Drawing for the job (mm, zero at the part's lowest x, y, z). A direction names the side the tool comes from. Round coordinates to 2 decimals unless told otherwise and drop trailing zeros. Write each loop counter-clockwise with the first axis right and the second up, starting at its lowest first coordinate (ties: lowest second). Pieces come first, ordered by that corner, then holes. Notation, with made-up numbers: (16.5, 46) -> (24.5, 46) arc R15 ccw to (24.5, 75) -> close; hole circle Ø5 at (63.25, 53.25). An arc over 180 degrees is marked (long way). One line per question, with ' | ' between items.
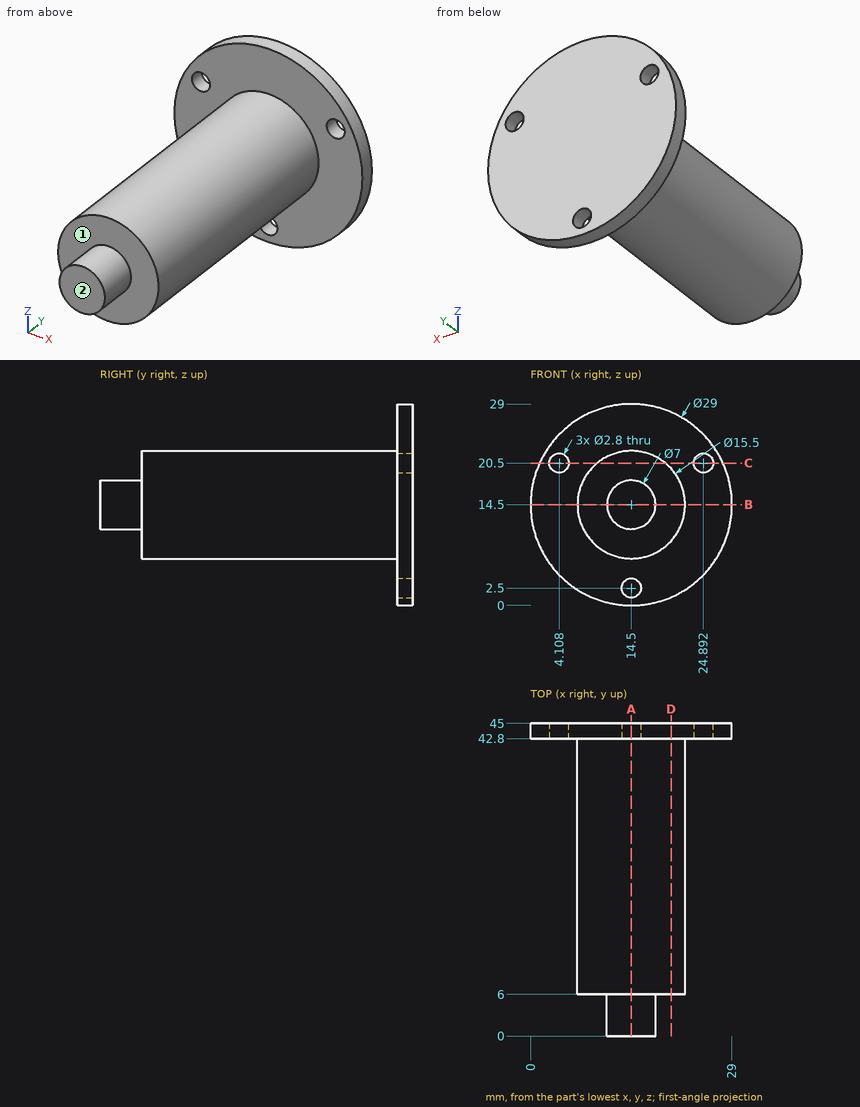
(1) Slice it at C-C (z = 20.5). Write the cut outline in (x, y) (1 decimal), then the cut area to 3 significant figures.
Calculated:
outline: (1.3, 42.8) -> (2.7, 42.8) -> (2.7, 45) -> (1.3, 45) -> close; (5.5, 42.8) -> (9.6, 42.8) -> (9.6, 6) -> (19.4, 6) -> (19.4, 42.8) -> (23.5, 42.8) -> (23.5, 45) -> (5.5, 45) -> close; (26.3, 42.8) -> (27.7, 42.8) -> (27.7, 45) -> (26.3, 45) -> close | area: 407 mm2
(2) 3-axis set-ups, long thin cutter, end or side, ignore diameter. For the marked faces 1 and 2: which of +Z, -Z, +X, -X, +Y, -Y reach the whole face in a straight line?
Calculated:
face 1: -Y | face 2: +Z, -Z, +X, -X, -Y
(3) Drop flat-ended pins along their axis: pin 1 (1.5 mm diameter, centred on x = 10, y = 14, fed in from +Z); pin 2 (3.5 mm diameter, centred on x = 14.5, z = 2.5, fed in from -Y); pin 3 (4 mm diameter, centred on x = 21.5, z = 14, fed in from -Y); pin 4 (17 mm diameter, centred on x = 11.5, z = 14, fed in from -Y). Give the stop position or say it passes through.
Calculated:
pin 1: z = 21.28 | pin 2: y = 42.8 | pin 3: y = 6 | pin 4: y = 0
(4) Wall check: line 1 (Z direction, x = 14.5, y = 43.4); line 2 (Y direction, x = 24.75, z = 16.75); line 3 (Y direction, x = 20.25, z = 10.75). Give the ranges that are in metal, low to high. Write a range as from..to.
Calculated:
line 1: 0..1.1, 3.9..29 | line 2: 42.8..45 | line 3: 6..45
(5) Slice it at A-A (x = 14.5). Write the cut outline in (y, z), then the cut area to 3 significant figures.
Calculated:
outline: (0, 11) -> (6, 11) -> (6, 6.75) -> (42.8, 6.75) -> (42.8, 3.9) -> (45, 3.9) -> (45, 29) -> (42.8, 29) -> (42.8, 22.25) -> (6, 22.25) -> (6, 18) -> (0, 18) -> close; (42.8, 0) -> (45, 0) -> (45, 1.1) -> (42.8, 1.1) -> close | area: 670 mm2
(6) Slice it at B-B (z = 14.5). Write the cut outline in (x, y).
Calculated:
outline: (0, 42.8) -> (6.75, 42.8) -> (6.75, 6) -> (11, 6) -> (11, 0) -> (18, 0) -> (18, 6) -> (22.25, 6) -> (22.25, 42.8) -> (29, 42.8) -> (29, 45) -> (0, 45) -> close
(7) Slice it at D-D (x = 20.25). Write the cut outline in (y, z).
Calculated:
outline: (6, 9.3) -> (42.8, 9.3) -> (42.8, 1.19) -> (45, 1.19) -> (45, 27.81) -> (42.8, 27.81) -> (42.8, 19.7) -> (6, 19.7) -> close
